Source: three-view drawing plus pictorial views. Frame: mm from the lowest corner of the part. Coordinates: 2 decimals unless noted, no trailing zeros. Loops run counter-clockwise (first coordinate to the right, second up) from the corner with the lowest first, then second, coordinate; pieces in that order, holes last. Notation, with made-up numbers: M 72,82.25 L 97,82.25 A14 ccw 97,107.25 Z; hole C 88.25,47 d4. An arc over 180 degrees is marked long. Use a Markdown table: item, result. Add a question column.
1. Pin query (flat end, axial travel): pin 1 (1.6 mm diameter, centred on x = 2.9, y = 79.3, fed in from -Z). Return the tip coordinate at first contact, or that it passes through.
2. Section D-D on z = 2.85. Output: boundary loops of the cut face in (x, y).
3. Draft query along X for the marked faces 1 and 2. Return one class per face: +X half, -X half, draft (parallel to the pull), parting line (faces both ways), or undercut.
4. Section C-C on x = 9. Output: boundary loops of the cut face in (y, z).
5. Section A-A on x = 47.5. Output: boundary loops of the cut face in (y, z), then the cut area to 3 significant figures.
6. Line query: L1, parallel to Y at x = 28.5, z = 1.9; L2, parallel to Y at x = 12.5, z = 0.8. Output: solid intervals per line, ascending. Write a range as [from, to].
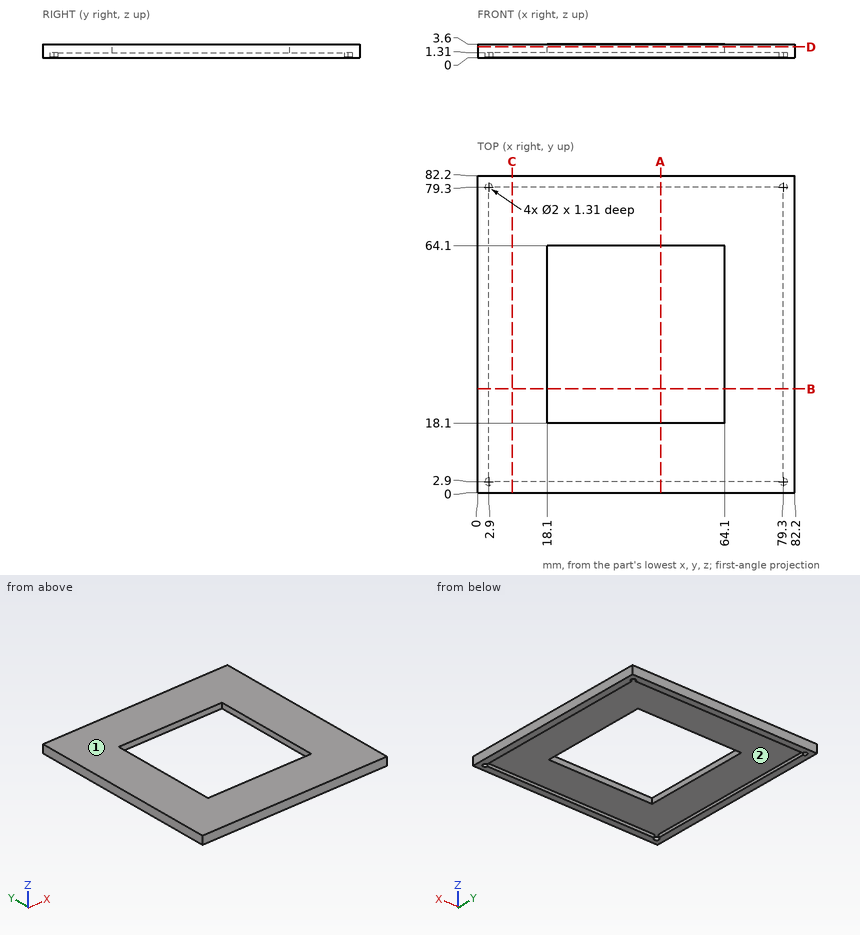
Answers below:
| question | item | result |
|---|---|---|
| 1 | pin 1 | stops at z = 1.31 |
| 2 | outline | M 0,0 L 82.2,0 L 82.2,82.2 L 0,82.2 Z; hole M 18.1,18.1 L 64.1,18.1 L 64.1,64.1 L 18.1,64.1 Z |
| 3 | face 1 | draft |
| 3 | face 2 | undercut |
| 4 | outline | M 0,0 L 2.9,0 L 2.9,1.31 L 79.3,1.31 L 79.3,0 L 82.2,0 L 82.2,3.6 L 0,3.6 Z |
| 5 | outline | M 0,0 L 2.9,0 L 2.9,1.31 L 18.1,1.31 L 18.1,3.6 L 0,3.6 Z; M 64.1,1.31 L 79.3,1.31 L 79.3,0 L 82.2,0 L 82.2,3.6 L 64.1,3.6 Z |
| 5 | area | 90.5 mm² |
| 6 | L1 | y = [0, 18.1], [64.1, 82.2] |
| 6 | L2 | y = [0, 2.9], [79.3, 82.2] |
